```python
from build123d import *

# Parameters (mm, degrees)
F0_W     = 511.175
F0_H     = 511.175
F1_DEPTH = 73.025
F2_W     = 584.2
F2_H     = 584.2
F2_W_2   = 511.175
F2_H_2   = 511.175
F3_DEPTH = 4.7625
F4_W     = 504.825
F4_H     = 504.825
F5_DEPTH = 77.7885


with BuildPart() as f1:
    # F0 (on Front) → F1 (new body)
    with BuildSketch(Plane.XZ):
        Rectangle(F0_W, F0_H)
    extrude(amount=-F1_DEPTH)

    # F2 (on face) → F3 (join)
    with BuildSketch(Plane.XZ):
        Rectangle(F2_W, F2_H)
        Rectangle(F2_W_2, F2_H_2, mode=Mode.SUBTRACT)
        Rectangle(F2_W_2, F2_H_2)
    extrude(amount=F3_DEPTH)

    # F4 (on face) → F5 (cut, through all)
    with BuildSketch(Plane.XZ.offset(4.7625)):
        Rectangle(F4_W, F4_H)
    extrude(amount=-F5_DEPTH, mode=Mode.SUBTRACT)


solid = f1.part
```
Part model, mm, in its own coordinate system. A direction names the side the tool comes from. Round coordinates to 2 decimals unless told otherwise and drop trailing zeros. Loops run counter-clockwise (first coordinate to the right, second up) from the corner with the lowest first, then second, coordinate; pieces in that order, holes last.
Item 1: Cut at A-A, the plane z = 138.5. Give the cut face in (x, y) (1 decimal).
Item 2: Drop flat-ended pins along their axis: P1, Ø3, axis at x = -176, y = 46, coming from the +Z side; P2, Ø2, axis at y = 59.5, z = -43, coming from the +X side; P3, Ø4, axis at y = 41.5, z = -209, coming from the -X side. Give the stop position or say it passes through.
Item 3: Drill centre lines: line 1 (X direction, y = -1, z = 137); line 2 (X direction, y = 21, z = -109.5). Where is each one in solid material? Low to high.
Item 4: Cut at C-C, the plane y = 27. Give the cut face in (x, z), then the cut area to 3 significant figures.
Item 5: 3-axis set-ups, long thin cutter, end or side, ignore diameter. For faces 5 (the face through (-264, -4.762, 4)), 6 (the face through (-4, 34, -252.412)), 7 (the face through (-4, 36, 255.588)), 8 (the face through (255.588, 36, -4)): which of +Z, -Z, +X, -X, +Y, -Y reach the whole face in a straight line?
Item 6: Cut at B-B, the plane x = -121.5. Give the cut face in (y, z) (1 decimal), then the cut area to 3 significant figures.
Item 7: Mould opens along X. For faces 1 (the face through (-4, 36, -255.588)), 2 (the face through (-255.588, 36, -4)), 3 (the face through (252.412, 34, -4)), 4 (the face through (-252.412, 34, -4)) say: +X half, -X half, draft (parallel to the pull), parting line (faces both ways), or undercut.
A:
1. outline: (-292.1, -4.8) - (-252.4, -4.8) - (-252.4, 73) - (-255.6, 73) - (-255.6, 0) - (-292.1, 0) - close; (252.4, -4.8) - (292.1, -4.8) - (292.1, 0) - (255.6, 0) - (255.6, 73) - (252.4, 73) - close
2. P1: stops at z = 255.59
2. P2: stops at x = 255.59
2. P3: stops at x = -255.59
3. line 1: x = -292.1 to -252.41, 252.41 to 292.1
3. line 2: x = -255.59 to -252.41, 252.41 to 255.59
4. outline: (-255.59, -255.59) - (255.59, -255.59) - (255.59, 255.59) - (-255.59, 255.59) - close; hole (-252.41, -252.41) - (252.41, -252.41) - (252.41, 252.41) - (-252.41, 252.41) - close
4. area: 6,450 mm2
5. face 5: +Z, -Z, +X, -X, -Y
5. face 6: +Y, -Y
5. face 7: +Z, +X, -X, +Y
5. face 8: +Z, -Z, +X, +Y
6. outline: (-4.8, -292.1) - (0, -292.1) - (0, -255.6) - (73, -255.6) - (73, -252.4) - (-4.8, -252.4) - close; (-4.8, 252.4) - (73, 252.4) - (73, 255.6) - (0, 255.6) - (0, 292.1) - (-4.8, 292.1) - close
6. area: 842 mm2
7. face 1: draft
7. face 2: -X half
7. face 3: undercut
7. face 4: undercut
